Source: CAD feature listing. Evaluate the final solid. Frame: model axes, mm. Coordinates: 2 decimals unless noted, no trailing zeros.
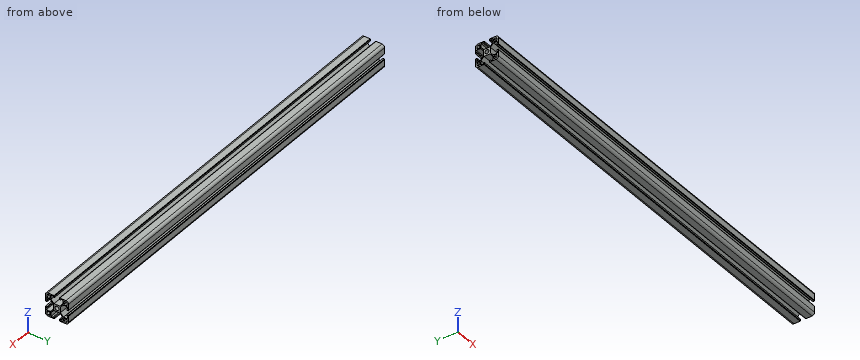
```python
from build123d import *

# Parameters (mm, degrees)
SKETCH1_R                 = 3.4
F_40_X_40L_X_R4_5_1_DEPTH = 750


with BuildPart() as part:
    # Sketch1 → 铝型材 40 X 40L X R4.5(1) (new body)
    with BuildSketch(Plane(origin=(-244.796828543, 0, 0), x_dir=(0, 0, -1), z_dir=(1, 0, 0))):
        with BuildLine():
            Line((-5.1, 20), (-5.1, 19.5))
            Line((-5.1, 19.5), (-4.1, 19.5))
            Line((-4.1, 19.5), (-4.1, 17))
            Line((-4.1, 17), (-6.1, 17))
            Line((-6.1, 17), (-6.1, 18.5))
            Line((-6.1, 18.5), (-10.3, 18.5))
            Line((-10.3, 18.5), (-10.3, 11.3))
            Line((-10.3, 11.3), (-5, 6))
            Line((-5, 6), (5, 6))
            Line((5, 6), (10.3, 11.3))
            Line((10.3, 11.3), (10.3, 18.5))
            Line((10.3, 18.5), (6.1, 18.5))
            Line((6.1, 18.5), (6.1, 17))
            Line((6.1, 17), (4.1, 17))
            Line((4.1, 17), (4.1, 19.5))
            Line((4.1, 19.5), (5.1, 19.5))
            Line((5.1, 19.5), (5.1, 20))
            Line((5.1, 20), (15.5, 20))
            ThreePointArc((15.5, 20), (18.681980515, 18.681980515), (20, 15.5))
            Line((20, 15.5), (20, 5.1))
            Line((20, 5.1), (19.5, 5.1))
            Line((19.5, 5.1), (19.5, 4.1))
            Line((19.5, 4.1), (17, 4.1))
            Line((17, 4.1), (17, 6.1))
            Line((17, 6.1), (18.5, 6.1))
            Line((18.5, 6.1), (18.5, 10.3))
            Line((18.5, 10.3), (11.3, 10.3))
            Line((11.3, 10.3), (6, 5))
            Line((6, 5), (6, -5))
            Line((6, -5), (11.3, -10.3))
            Line((11.3, -10.3), (18.5, -10.3))
            Line((18.5, -10.3), (18.5, -6.1))
            Line((18.5, -6.1), (17, -6.1))
            Line((17, -6.1), (17, -4.1))
            Line((17, -4.1), (19.5, -4.1))
            Line((19.5, -4.1), (19.5, -5.1))
            Line((19.5, -5.1), (20, -5.1))
            Line((20, -5.1), (20, -15.5))
            ThreePointArc((20, -15.5), (18.681980515, -18.681980515), (15.5, -20))
            Line((15.5, -20), (5.1, -20))
            Line((5.1, -20), (5.1, -19.5))
            Line((5.1, -19.5), (4.1, -19.5))
            Line((4.1, -19.5), (4.1, -17))
            Line((4.1, -17), (6.1, -17))
            Line((6.1, -17), (6.1, -18.5))
            Line((6.1, -18.5), (10.3, -18.5))
            Line((10.3, -18.5), (10.3, -11.3))
            Line((10.3, -11.3), (5, -6))
            Line((5, -6), (-5, -6))
            Line((-5, -6), (-10.3, -11.3))
            Line((-10.3, -11.3), (-10.3, -18.5))
            Line((-10.3, -18.5), (-6.1, -18.5))
            Line((-6.1, -18.5), (-6.1, -17))
            Line((-6.1, -17), (-4.1, -17))
            Line((-4.1, -17), (-4.1, -19.5))
            Line((-4.1, -19.5), (-5.1, -19.5))
            Line((-5.1, -19.5), (-5.1, -20))
            Line((-5.1, -20), (-15.5, -20))
            ThreePointArc((-15.5, -20), (-18.681980515, -18.681980515), (-20, -15.5))
            Line((-20, -15.5), (-20, -5.1))
            Line((-20, -5.1), (-19.5, -5.1))
            Line((-19.5, -5.1), (-19.5, -4.1))
            Line((-19.5, -4.1), (-17, -4.1))
            Line((-17, -4.1), (-17, -6.1))
            Line((-17, -6.1), (-18.5, -6.1))
            Line((-18.5, -6.1), (-18.5, -10.3))
            Line((-18.5, -10.3), (-11.3, -10.3))
            Line((-11.3, -10.3), (-6, -5))
            Line((-6, -5), (-6, 5))
            Line((-6, 5), (-11.3, 10.3))
            Line((-11.3, 10.3), (-18.5, 10.3))
            Line((-18.5, 10.3), (-18.5, 6.1))
            Line((-18.5, 6.1), (-17, 6.1))
            Line((-17, 6.1), (-17, 4.1))
            Line((-17, 4.1), (-19.5, 4.1))
            Line((-19.5, 4.1), (-19.5, 5.1))
            Line((-19.5, 5.1), (-20, 5.1))
            Line((-20, 5.1), (-20, 15.5))
            ThreePointArc((-20, 15.5), (-18.681980515, 18.681980515), (-15.5, 20))
            Line((-15.5, 20), (-5.1, 20))
        make_face()
        Circle(SKETCH1_R, mode=Mode.SUBTRACT)
        with BuildLine():
            Line((11.8, 17.5), (15, 17.5))
            ThreePointArc((15, 17.5), (16.767766953, 16.767766953), (17.5, 15))
            Line((17.5, 15), (17.5, 11.8))
            Line((17.5, 11.8), (11.8, 11.8))
            Line((11.8, 11.8), (11.8, 17.5))
        make_face(mode=Mode.SUBTRACT)
        with BuildLine():
            Line((-15, 17.5), (-11.8, 17.5))
            Line((-11.8, 17.5), (-11.8, 11.8))
            Line((-11.8, 11.8), (-17.5, 11.8))
            Line((-17.5, 11.8), (-17.5, 15))
            ThreePointArc((-17.5, 15), (-16.767766953, 16.767766953), (-15, 17.5))
        make_face(mode=Mode.SUBTRACT)
        with BuildLine():
            Line((-17.5, -11.8), (-11.8, -11.8))
            Line((-11.8, -11.8), (-11.8, -17.5))
            Line((-11.8, -17.5), (-15, -17.5))
            ThreePointArc((-15, -17.5), (-16.767766953, -16.767766953), (-17.5, -15))
            Line((-17.5, -15), (-17.5, -11.8))
        make_face(mode=Mode.SUBTRACT)
        with BuildLine():
            Line((11.8, -11.8), (17.5, -11.8))
            Line((17.5, -11.8), (17.5, -15))
            ThreePointArc((17.5, -15), (16.767766953, -16.767766953), (15, -17.5))
            Line((15, -17.5), (11.8, -17.5))
            Line((11.8, -17.5), (11.8, -11.8))
        make_face(mode=Mode.SUBTRACT)
    extrude(amount=F_40_X_40L_X_R4_5_1_DEPTH)


solid = part.part
```
Q1. Pin query (flat end, axial travel): P1, Ø6, axis at x = 45.5, z = 0, coming from the +Y side; P2, Ø0.5, axis at x = -8, y = 4.5, coming from the +Z side; P3, Ø4, axis at x = 45, y = -2, coming from the -Z side; P4, Ø11, axis at x = 254, y = -0.5, coming from the -Z side. Return the tip coordinate at first contact, or that it passes through.
Solutions:
P1: stops at y = 6
P2: stops at z = 19.5
P3: stops at z = -6
P4: stops at z = -20
Q2. Section query A-A on x = -53. Give the number of separate pieces and of enclosed holes in the cut face, plus the area to 3 significant figures.
Solutions:
separate pieces: 1
enclosed holes: 5
area: 475 mm2
Q3. Material intervals for line 1 along Y through (x, z) = (-27.5, 15.5); line 2 along Z through (x, y) = (8, 13), sorted ascending.
Solutions:
line 1: y = -20 to -17.45, -11.8 to -10.3, 10.3 to 11.8, 17.45 to 20
line 2: z = -20 to -17.5, -11.8 to -10.3, 10.3 to 11.8, 17.5 to 20
